Read the model definition and answer for the solid it produces. Units are mm, in the model's axes. A direction names the side the tool comes from. Coordinates: 2 decimals unless noted, no trailing zeros. Order: outer loops, then holes, each group sorted by start corner. A loop starts at its lowest first (then second) coordinate and runs counter-clockwise, first axis right, second up. Notation, with made-up numbers: M 39,70.25 L 88,70.25 A17 cw 88,98.25 Z; hole C -13.75,9 d11. An arc over 180 degrees is marked long. Put each result on its own line as item: value.
Autodesk Inventor part; units mm, degrees
ref_plane "YZ Plane" through (0, 0, 0) normal (1, 0, 0) x (0, 1, 0)
ref_plane "XZ Plane" through (0, 0, 0) normal (0, 1, 0) x (-1, 0, 0)
ref_plane "XY Plane" through (0, 0, 0) normal (0, 0, 1) x (1, 0, 0)
sketch "Sketch1" plane through (0, 0, 0) normal (0, 1, 0) x (-1, 0, 0)
  line L0 (0, -2.5) -> (-6.25, -2.5)
  line L1 (-6.25, -2.5) -> (-8.75, -4)
  line L2 (-8.75, -4) -> (-8.75, 4)
  line L3 (-8.75, 4) -> (-6.25, 2.5)
  line L4 (-6.25, 2.5) -> (0, 2.5)
  line L5 (0, 2.5) -> (0, -2.5)
  line L6 (0, -5) -> (-11.25, -5)
  line L7 (-11.25, -5) -> (-11.25, 5)
  line L8 (-11.25, 5) -> (0, 5)
  line L9 (0, 5) -> (0, -5)
  point P0 (-8.75, 0)
  point P1 (0, 0)
  point P2 (0, 0)
  point P3 (0, 2.5)
  dimension "d16" = 5
  dimension "d17" = 2.5
  dimension "d18" = 8
  dimension "d19" = 8.75
  dimension "d20" = 11.25
  dimension "d21" = 5
  dimension "d22" = 5
extrude "Extrusion1" add sketch "Sketch1" along normal blind 3
extrude "Extrusion2" add sketch "Sketch1" along normal blind 80 contours L0 L1 L2 L3 L4 L5
mirror "Mirror1" about plane through (0, 0, -5) normal (-1, 0, 0) of "Extrusion1", "Extrusion2"
properties part number "drawerconnector"
Q1. Find section B-B on y = 47. Write down the section's boundary in (x, z), plus the area to 3 significant figures.
Answers below:
outline: M -8.75,-4 L -6.25,-2.5 L 6.25,-2.5 L 8.75,-4 L 8.75,4 L 6.25,2.5 L -6.25,2.5 L -8.75,4 Z
area: 95.0 mm^2
Q2. Consider line 1 along Z through (x, y) = (-4.5, 46.5); line 2 along Y through (x, z) = (6, 4.25); line 3 along X through (y, z) = (30.5, 1). Determine where each line is inside the solid, lowest interval first.
Answers below:
line 1: z = -2.5 to 2.5
line 2: y = 0 to 3
line 3: x = -8.75 to 8.75
Q3. For a pull along X with two mould halves and no side action, classify faces 1 (the face through (-8.75, 41, 0)), 2 (the face through (7.52, 40.96, 3.26)), 3 (the face through (0, 80, 0)), 4 (the face through (11.25, 1, 0)) as +X half, -X half, draft (parallel to the pull), parting line (faces both ways), or undercut.
Answers below:
face 1: -X half
face 2: undercut
face 3: draft
face 4: +X half
Q4. A tool of negligible diameter and unlimited length cuts with its end or side. For faces 5 (the face through (8.75, 41, 0)), 6 (the face through (0, 0, 0)), 7 (the face through (-7.52, 40.96, -3.26)), 8 (the face through (-7.48, 40.96, 3.24)), from which of +Z, -Z, +X, -X, +Y, -Y can it reach the whole face along a straight path? Write none if from no direction.
Answers below:
face 5: +Z, -Z, +X, +Y
face 6: +Z, -Z, +X, -X, -Y
face 7: -Z, +Y
face 8: +Z, +Y
Q5. Find section A-A on x = 8. Write down the section's boundary in (y, z), plus the area to 3 significant figures.
Answers below:
outline: M 0,-5 L 3,-5 L 3,-3.55 L 80,-3.55 L 80,3.55 L 3,3.55 L 3,5 L 0,5 Z
area: 577 mm^2
Q6. Given pin 1 (5 mm diameter, centred on y = 46, z = 1.5, fed in from +X); pin 2 (6 mm diameter, centred on x = 1.5, y = 24, fed in from +Z); pin 3 (1 mm diameter, centred on y = 50, z = 0, fed in from -X), each flat-ended and moving along its own axis, determine where each tip first touches the part or whether it passes through.
Answers below:
pin 1: stops at x = 8.75
pin 2: stops at z = 2.5
pin 3: stops at x = -8.75
